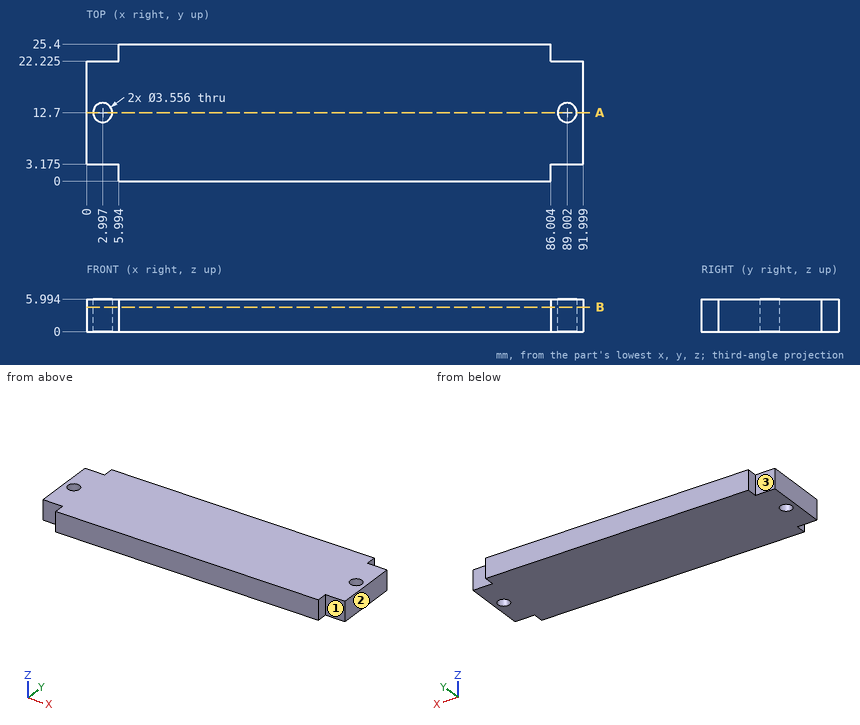
Source: three-view drawing plus pictorial views. Frame: mm from the lowest corner of the part. A direction names the side the tool comes from. Round coordinates to 2 decimals unless told otherwise and drop trailing zeros. Order: outer loops, then holes, each group sorted by start corner. A loop starts at its lowest first (then second) coordinate and runs counter-clockwise, first axis right, second up. Notation, with made-up numbers: (81, 80.25) -> (117, 80.25) arc R28 cw to (117, 105.25) -> close; hole circle Ø7 at (-38, -13). An arc over 180 degrees is marked (long way). Use one line per item in the form item = value.
(1) Access query for the marked faces 1, 2 and 3. Directions: +Z, -Z, +X, -X, +Y, -Y. A direction counts if a zero-diameter tool reaches every point of the face in a straight line with its end or side. Return the directions, or none.
Results list:
face_1 = +Z, -Z, +X, -Y
face_2 = +Z, -Z, +X, +Y, -Y
face_3 = +Z, -Z, -X, +Y
(2) Ray query, probe 1 along X at (y, z) = (14, 0.6) (1 decimal). Return the intervals inside material, ascending. Write a range as [from, to].
Results list:
probe_1 = [0, 1.8], [4.2, 87.8], [90.2, 92]
(3) Section A-A on y = 12.7. Return loops of the section in (x, z) (1 decimal), and give its area (3 significant figures).
Results list:
outline = (0, 0) -> (1.2, 0) -> (1.2, 6) -> (0, 6) -> close; (4.8, 0) -> (87.2, 0) -> (87.2, 6) -> (4.8, 6) -> close; (90.8, 0) -> (92, 0) -> (92, 6) -> (90.8, 6) -> close
area = 509 mm^2
(4) First-contact query: pin 1 Ø3 at (x, z) = (88, 3.5) entering from +Y (3 decimals); pin 2 Ø1 at (y, z) = (1, 3) entering from +X; pin 3 Ø1.8 at (x, z) = (4, 3) entering from -Y (3 decimals). Flat tips, straight axial feed; report the tip coordinate or a pass-through.
Results list:
pin_1 = 22.225
pin_2 = 86
pin_3 = 3.175
(5) Section B-B on z = 4.5. Return loops of the section in (x, y) (1 decimal), and give its area (3 significant figures).
Results list:
outline = (0, 3.2) -> (6, 3.2) -> (6, 0) -> (86, 0) -> (86, 3.2) -> (92, 3.2) -> (92, 22.2) -> (86, 22.2) -> (86, 25.4) -> (6, 25.4) -> (6, 22.2) -> (0, 22.2) -> close; hole circle Ø3.6 at (3, 12.7); hole circle Ø3.6 at (89, 12.7)
area = 2,240 mm^2
